Can you work these out from the model? Positions are in its coordinate system, mm. Give positions to 0.01 mm unless a question says otherwise; leave off trailing zeros. Order: outer loops, then holes, each group sorted by start corner. A loop starts at its lowest first (then second) coordinate and runs counter-clockwise, first axis right, second up.
Item 1: I'm going to push a flat-ended pin straight in: pin 1 Ø2.5 at (x, y) = (29.5, 6.5) entering from +Z. Where does the tip first touch, or does it pass through?
Item 2: I want a section at A-A, the plane x = 53. Write out the boundary of the cut face in (y, z).
Item 3: I want a section at C-C, the plane y = 38. Write out the boundary of the cut face in (x, z).
Item 4: I want a section at B-B, the plane z = 4.25. Write out the boundary of the cut face in (x, y).
Item 5: If I drill on line 1 along Y through (x, z) = (73, 3.75); line 2 along X through (y, z) = (9, 3); line 3 along Z through (x, y) = (4.5, 2.5), over which ranges is the centre line in solid material (lowest first)?
```python
from build123d import *

# Parameters (mm, degrees)
BOSS_EXTRUDE1_DEPTH     = 57.15
SKETCH2_W               = 2.9972
SKETCH2_H               = 3.2512
CUT_EXTRUDE1_DEPTH      = 82.0006
CUT_EXTRUDE1_DEPTH_BACK = 1


with BuildPart() as part:
    # Sketch1 → Boss-Extrude1 (new body)
    with BuildSketch(Plane(origin=(0, 0, 0), x_dir=(1, 0, 0), z_dir=(0, 1, 0))):
        Polygon((0, 0), (81.0006, 0), (74.6506, -6.35), (6.35, -6.35), align=None)
    extrude(amount=BOSS_EXTRUDE1_DEPTH)

    # Sketch2 → Cut-Extrude1 (cut, two sides)
    with BuildSketch(Plane(origin=(0, 0, 0), x_dir=(0, 0, -1), z_dir=(1, 0, 0))) as cut_extrude1_sk:
        with Locations((-4.8514, 6.3881)):
            Rectangle(SKETCH2_W, SKETCH2_H)
    extrude(amount=CUT_EXTRUDE1_DEPTH, mode=Mode.SUBTRACT)
    extrude(cut_extrude1_sk.sketch, amount=-CUT_EXTRUDE1_DEPTH_BACK, mode=Mode.SUBTRACT)


solid = part.part
```
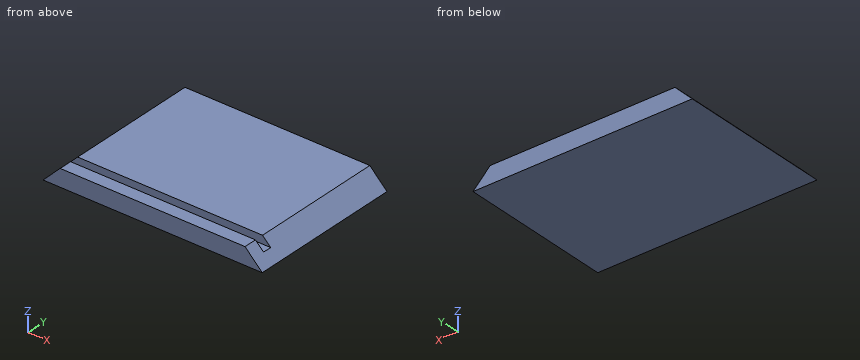
Results list:
1. pin 1: stops at z = 3.35
2. outline: (0, 0) - (57.15, 0) - (57.15, 6.35) - (8.01, 6.35) - (8.01, 3.35) - (4.76, 3.35) - (4.76, 6.35) - (0, 6.35) - close
3. outline: (0, 0) - (81, 0) - (74.65, 6.35) - (6.35, 6.35) - close
4. outline: (4.25, 0) - (76.75, 0) - (76.75, 4.76) - (4.25, 4.76) - close; (4.25, 8.01) - (76.75, 8.01) - (76.75, 57.15) - (4.25, 57.15) - close
5. line 1: y = 0 to 4.76, 8.01 to 57.15
5. line 2: x = 3 to 78
5. line 3: z = 0 to 4.5
